Verification items for the finished model (mm, model axes). Face numbers are marked on the shaded views. A direction names the side the tool comes from. Coordinates: 2 decimals unless noted, no trailing zeros. Loops run counter-clockwise (first coordinate to the right, second up) from the corner with the lowest first, then second, coordinate; pieces in that order, holes last.
Q1. Material ranges on probe 1 along X at (y, z) = (21.75, -1.5); probe 2 along Z at (x, y) = (-13.5, 24) (3 decimals); probe 3 along X at (y, z) = (10.5, -9.5), recorded low to high.
Q2. Go/stop test with flat-tipped pins: P1, Ø6, axis at y = 26, z = -14, coming from the -X side; P2, Ø8, axis at y = 26, z = -22.5, coming from the -X side; P3, Ø3, axis at x = -0.5, y = 18.5, coming from the -Z side. Record where each tip stops, or that it passes through.
Q3. Sectioned sample at B-B (y = 19.5). Enter the section's corners in (x, z) (3 decimals).
Q4. Access from +Z, -Z, +X, -X, +Y, -Y to the whole of each face (thin tool, end or side, straight path). Record for the marked faces 1, 2, 3, 4 and 5.
Q5. Sectioned sample at C-C (y = 2). Enter the section's corners in (x, z) (3 decimals), then the cut area to 3 significant figures.
Q6. Sectioned sample at D-D (x = 2.5). Enter the section's corners in (y, z) (3 decimals).
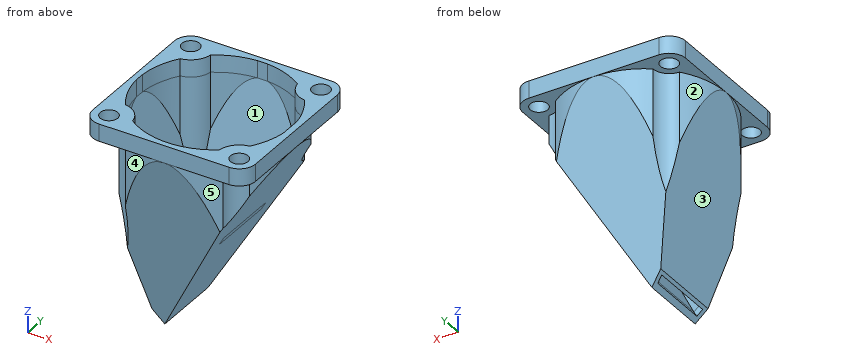
```python
from build123d import *

# Parameters (mm, degrees)
F0_R          = 15
F1_DEPTH      = 50.8
F3_DEPTH      = 50.8
F5_DEPTH      = 16
F5_DEPTH_BACK = 25.4
F6_R          = 2.999994
F7_DEPTH      = 75
F8_T          = -1.0294366
F9_R          = 1.625
F10_DEPTH     = 3.175
F11_R         = 2.999994
F12_W         = 12.402147986
F12_H         = 1.7178952694
F13_DEPTH     = 1.0294366
F15_REACH     = 37.7778044783
F16_DEPTH     = 1.7178952694


# Not quite as in the source:
# - an extrude ends at something that could not be found from the text; its depth is read off the source's solid


with BuildPart() as f1:
    # F0 (on Top) → F1 (new body)
    with BuildSketch(Plane.XY):
        with Locations((0, 15)):
            Circle(F0_R)
    extrude(amount=-F1_DEPTH)

    # F2 (on Front) → F3 (cut)
    with BuildSketch(Plane.XZ):
        Polygon((-15, 0), (-15, -50.8), (15, -50.8), (15, 0), (-5.2591228073, -36.0019072397), (-7.2556595325, -33.5332099912), align=None)
    extrude(amount=-F3_DEPTH, mode=Mode.SUBTRACT)

    # F4 (on Right) → F5 (cut, two sides)
    with BuildSketch(Plane.YZ) as f5_sk:
        Polygon((30, -36.0019072397), (30, 0), (21.35, -36.0019072397), align=None)
        Polygon((8.65, -36.0019072397), (0, 0), (0, -36.0019072397), align=None)
    extrude(amount=-F5_DEPTH, mode=Mode.SUBTRACT)
    extrude(f5_sk.sketch, amount=F5_DEPTH_BACK, mode=Mode.SUBTRACT)

    # F6 (on face) → F7 (cut, through all)
    with BuildSketch(Plane.XY):
        with Locations((12.000006, 27.000006)):
            Circle(F6_R)
        with Locations((12.000006, 2.999994)):
            Circle(F6_R)
        with Locations((-12.000006, 2.999994)):
            Circle(F6_R)
        with Locations((-12.000006, 27.000006)):
            Circle(F6_R)
    extrude(amount=-F7_DEPTH, mode=Mode.SUBTRACT)

    # F8
    f8_openings = [f1.faces().sort_by_distance(p)[0] for p in [
        (0, 15, 0),
    ]]
    offset(amount=F8_T, openings=f8_openings)

    # F9 (on face) → F10 (join)
    with BuildSketch(Plane.XY):
        with BuildLine():
            Line((1.23e-08, 0), (15, 0))
            Line((15, 0), (15, 15))
            ThreePointArc((15, 15), (14.230247099, 10.2565763946), (11.999991, 5.999988))
            ThreePointArc((11.999991, 5.999988), (9.8786898991, 5.1213101009), (9.000012, 3.000009))
            ThreePointArc((9.000012, 3.000009), (4.7434236112, 0.7697529029), (1.23e-08, 0))
        make_face()
        with Locations((12.000006, 2.999994)):
            Circle(F9_R, mode=Mode.SUBTRACT)
        with BuildLine():
            Line((-15, 0), (1.23e-08, 0))
            ThreePointArc((1.23e-08, 0), (-4.7434235996, 0.769752899), (-9.000012, 3.000009))
            ThreePointArc((-9.000012, 3.000009), (-9.8786898991, 5.1213101009), (-11.999991, 5.999988))
            ThreePointArc((-11.999991, 5.999988), (-14.230247099, 10.2565763946), (-15, 15))
            Line((-15, 15), (-15, 0))
        make_face()
        with Locations((-12.000006, 2.999994)):
            Circle(F9_R, mode=Mode.SUBTRACT)
        with BuildLine():
            ThreePointArc((-9.000012, 3.000009), (-4.7434235996, 0.769752899), (1.23e-08, 0))
            ThreePointArc((1.23e-08, 0), (4.7434236112, 0.7697529029), (9.000012, 3.000009))
            ThreePointArc((9.000012, 3.000009), (9.8786898991, 5.1213101009), (11.999991, 5.999988))
            ThreePointArc((11.999991, 5.999988), (14.230247099, 10.2565763946), (15, 15))
            ThreePointArc((15, 15), (14.230247099, 19.7434236054), (11.999991, 24.000012))
            ThreePointArc((11.999991, 24.000012), (9.8786898991, 24.8786898991), (9.000012, 26.999991))
            ThreePointArc((9.000012, 26.999991), (4.7434236018, 29.2302471002), (-7.6e-09, 30))
            ThreePointArc((-7.6e-09, 30), (-4.743423609, 29.2302470978), (-9.000012, 26.999991))
            ThreePointArc((-9.000012, 26.999991), (-9.8786898991, 24.8786898991), (-11.999991, 24.000012))
            ThreePointArc((-11.999991, 24.000012), (-14.230247099, 19.7434236054), (-15, 15))
            ThreePointArc((-15, 15), (-14.230247099, 10.2565763946), (-11.999991, 5.999988))
            ThreePointArc((-11.999991, 5.999988), (-9.8786898991, 5.1213101009), (-9.000012, 3.000009))
        make_face()
        with BuildLine():
            Line((0.9042769799, 1.0587330254), (-0.9042769799, 1.0587330254))
            ThreePointArc((-0.9042769799, 1.0587330254), (-4.6276702262, 1.8181446681), (-8.0086800871, 3.5528307003))
            ThreePointArc((-8.0086800871, 3.5528307003), (-9.1507682984, 5.8492317016), (-11.4471692997, 6.9913199129))
            ThreePointArc((-11.4471692997, 6.9913199129), (-13.1875845683, 10.3886818623), (-13.9434671073, 14.1303065241))
            Line((-13.9434671073, 14.1303065241), (-13.9434671073, 15.8696934759))
            ThreePointArc((-13.9434671073, 15.8696934759), (-13.1875845683, 19.6113181377), (-11.4471692997, 23.0086800871))
            ThreePointArc((-11.4471692997, 23.0086800871), (-9.1507682984, 24.1507682984), (-8.0086800871, 26.4471692997))
            ThreePointArc((-8.0086800871, 26.4471692997), (-4.6276702262, 28.1818553319), (-0.9042769799, 28.9412669746))
            Line((-0.9042769799, 28.9412669746), (0.9042769799, 28.9412669746))
            ThreePointArc((0.9042769799, 28.9412669746), (4.6276702262, 28.1818553319), (8.0086800871, 26.4471692997))
            ThreePointArc((8.0086800871, 26.4471692997), (9.1507682984, 24.1507682984), (11.4471692997, 23.0086800871))
            ThreePointArc((11.4471692997, 23.0086800871), (12.9790918545, 20.1691214289), (13.8187656408, 17.053864133))
            Line((13.8187656408, 17.053864133), (13.8187656408, 12.946135867))
            ThreePointArc((13.8187656408, 12.946135867), (12.9790918545, 9.8308785711), (11.4471692997, 6.9913199129))
            ThreePointArc((11.4471692997, 6.9913199129), (9.1507682984, 5.8492317016), (8.0086800871, 3.5528307003))
            ThreePointArc((8.0086800871, 3.5528307003), (4.6276702262, 1.8181446681), (0.9042769799, 1.0587330254))
        make_face(mode=Mode.SUBTRACT)
        with BuildLine():
            ThreePointArc((11.999991, 24.000012), (14.230247099, 19.7434236054), (15, 15))
            Line((15, 15), (15, 30))
            Line((15, 30), (-7.6e-09, 30))
            ThreePointArc((-7.6e-09, 30), (4.7434236018, 29.2302471002), (9.000012, 26.999991))
            ThreePointArc((9.000012, 26.999991), (9.8786898991, 24.8786898991), (11.999991, 24.000012))
        make_face()
        with Locations((12.000006, 27.000006)):
            Circle(F9_R, mode=Mode.SUBTRACT)
        with BuildLine():
            Line((-15, 30), (-15, 15))
            ThreePointArc((-15, 15), (-14.230247099, 19.7434236054), (-11.999991, 24.000012))
            ThreePointArc((-11.999991, 24.000012), (-9.8786898991, 24.8786898991), (-9.000012, 26.999991))
            ThreePointArc((-9.000012, 26.999991), (-4.743423609, 29.2302470978), (-7.6e-09, 30))
            Line((-7.6e-09, 30), (-15, 30))
        make_face()
        with Locations((-12.000006, 27.000006)):
            Circle(F9_R, mode=Mode.SUBTRACT)
    extrude(amount=F10_DEPTH)

    # F11
    f11_edges = [f1.edges().sort_by_distance(p)[0] for p in [
        (15, 0, 1.5875),
        (-15, 0, 1.5875),
        (-15, 30, 1.5875),
        (15, 30, 1.5875),
    ]]
    fillet(f11_edges, radius=F11_R)

    # F12 (on face) → F13 (cut, through all)
    with BuildSketch(Plane(origin=(11.3924813609, 0, -6.4108181112), x_dir=(0, 1, 0), z_dir=(0.8714922589, 0, -0.4904092603))):
        with Locations((14.4248786382, -12.1594956145)):
            Rectangle(F12_W, F12_H)
    extrude(amount=-F13_DEPTH, mode=Mode.SUBTRACT)

    f15_end = f1.faces().sort_by_distance((-6.2722387902, 15, -34.7491996848))[0]
    # F14 (on face) → F15 (cut, up to a face of the model that its end follows)
    with BuildSketch(Plane(origin=(-6.3843651243, 0, -11.3454725151), x_dir=(0.8714922589, 0, -0.4904092603), z_dir=(0.4904092603, 0, 0.8714922589))):
        Polygon((12.0429472841, 9.2698510415), (12.0429472841, 20.7301489585), (10.7223677877, 20.9956137981), (10.7223677877, 9.0043862019), align=None)
    f15_long = extrude(amount=-F15_REACH, mode=Mode.PRIVATE)
    add(split(f15_long, bisect_by=f15_end, keep=Keep.BOTTOM, mode=Mode.PRIVATE), mode=Mode.SUBTRACT)

    # F16 (add, through all): a face of the model
    f16_faces = [f1.faces().sort_by_distance(p)[0] for p in [
        (4.5595432226, 14.4248786382, -17.5038680055),
    ]]
    extrude(f16_faces, amount=F16_DEPTH)


solid = f1.part
```
Geometry check:
1. probe 1: x = -13.4 to -12.23, 12.23 to 13.4
1. probe 2: z = 0 to 3.175
1. probe 3: x = -12.81 to -11.75, 8.47 to 9.65
2. P1: stops at x = -12.21
2. P2: stops at x = -10.64
2. P3: stops at z = -30.21
3. outline: (-15, 0) - (-14.309, 0) - (-14.309, -2.992) - (-7.256, -33.533) - (-6.849, -34.036) - (-6.306, -33.07) - (-13.226, -3.107) - (-13.226, 3.175) - (-15, 3.175) - close; (-5.956, -35.141) - (-5.259, -36.002) - (14.309, -1.228) - (14.309, 0) - (15, 0) - (15, 3.175) - (13.226, 3.175) - (13.226, -1.053) - close
4. face 1: +Z
4. face 2: -Z, -X, +Y
4. face 3: -Z, -X, +Y, -Y
4. face 4: -Z, -X, -Y
4. face 5: -Z, +X, -Y
5. outline: (-14.828, 0) - (-13.281, 0) - (-13.281, 3.175) - (-14.828, 3.175) - close; (-10.719, 0) - (-7.483, 0) - (-7.483, -8.324) - (7.483, -8.324) - (7.483, 0) - (10.719, 0) - (10.719, 3.175) - (5.116, 3.175) - (5.116, -3.918) - (-5.116, -3.918) - (-5.116, 3.175) - (-10.719, 3.175) - close; (13.281, 0) - (14.828, 0) - (14.828, 3.175) - (13.281, 3.175) - close
5. area: 130 mm2
6. outline: (0, 0) - (0.21, 0) - (0.21, -0.873) - (5.337, -22.213) - (24.663, -22.213) - (29.79, -0.873) - (29.79, 0) - (30, 0) - (30, 3.175) - (28.745, 3.175) - (28.745, -0.817) - (24.109, -20.114) - (5.891, -20.114) - (1.255, -0.817) - (1.255, 3.175) - (0, 3.175) - close
